Part print with two shaded views. Sizes in mm from the minimum x, y, z corner. A direction names the side the tool comes from. Coordinates: 2 decimals unless noted, no trailing zeros. Order: outer loops, then holes, each group sorted by start corner. A loop starts at its lowest first (then second) coordinate and runs counter-clockwise, first axis right, second up. Notation, with made-up numbers: (8.25, 89.25) - (39.25, 89.25) arc R19 cw to (39.25, 115.25) - close; hole circle Ø9 at (73, 49). An arc over 180 degrees is marked (long way). Return JSON: item names as keys, results as strings.
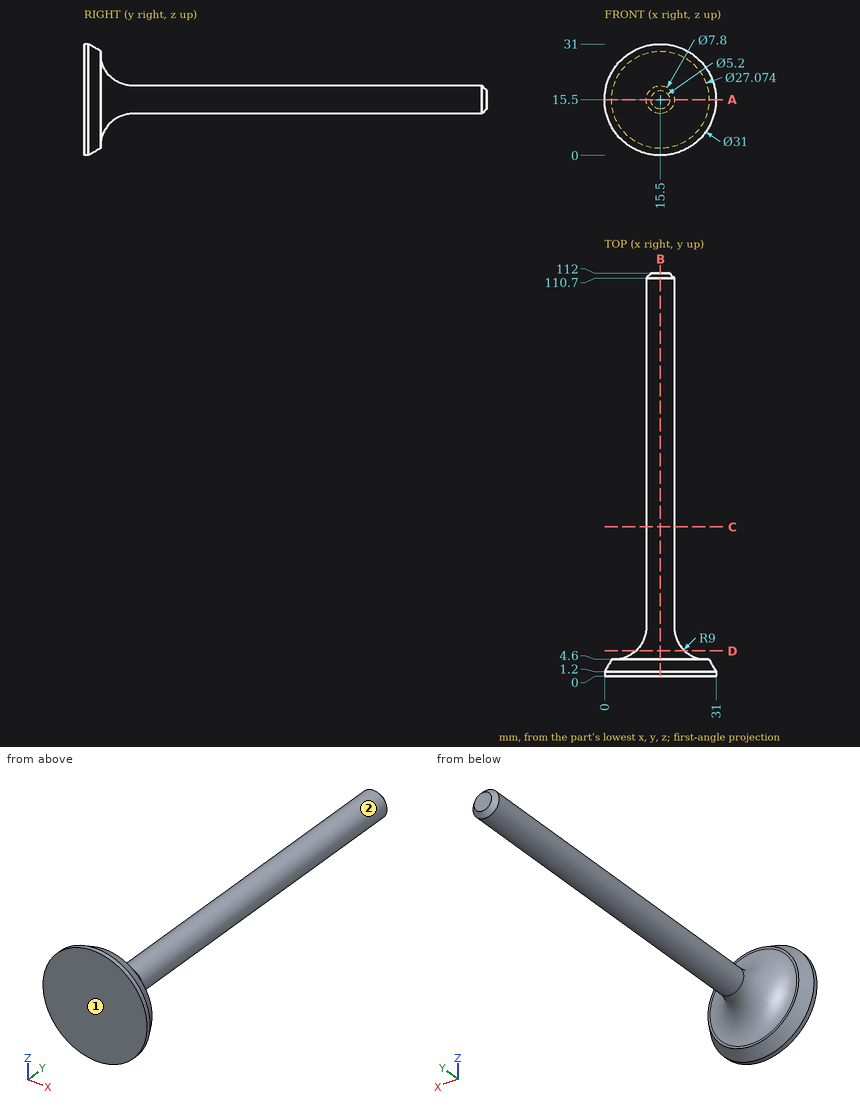
Item 1: Which spindle directions (+Z, -Z, +X, -X, +Y, -Y) get a long thin tool onto all of the face, cutting with end or side? Do the marked faces 1 and 2. Say none if no direction does.
Findings below:
{"face 1": "+Z, -Z, +X, -X, -Y", "face 2": "+Y"}
Item 2: Drop flat-ended pins along their axis: P1, Ø1.5, axis at x = 12, z = 7, coming from the +Y side; P2, Ø12, axis at x = 13, y = 21, coming from the -Z side; P3, Ø3, axis at x = 15.5, z = 10.5, coming from the +Y side; P4, Ø4, axis at y = 94.5, z = 9.5, coming from the +X side. Give the stop position or say it passes through.
Findings below:
{"P1": "stops at y = 5.78", "P2": "stops at z = 11.6", "P3": "stops at y = 111.1", "P4": "passes through"}
Item 3: Band-saw the part on B-B, the plane x = 15.5. List the corners of the cut face in (y, z).
Findings below:
{"outline": "(0, 0) - (1.2, 0) - (4.6, 1.96) - (4.6, 2.6) arc R9 cw to (13.6, 11.6) - (110.7, 11.6) - (112, 12.9) - (112, 18.1) - (110.7, 19.4) - (13.6, 19.4) arc R9 cw to (4.6, 28.4) - (4.6, 29.04) - (1.2, 31) - (0, 31) - close"}
Item 4: Band-saw the part on C-C, the plane y = 41.5. List the corners of the cut face in (x, z), then the cut area to 3 significant figures.
Findings below:
{"outline": "circle Ø7.8 at (15.5, 15.5)", "area": "47.8 mm²"}
Item 5: Wall check: L1, parallel to Y at x = 3, z = 19.5; L2, parallel to Y at x = 14.5, z = 26; L3, parallel to X at y = 61, z = 18. Give the ranges that are in metal, low to high. Write a range as [from, to].
Findings below:
{"L1": "y = [0, 4.6]", "L2": "y = [0, 4.91]", "L3": "x = [12.51, 18.49]"}
Item 6: Band-saw the part on D-D, the plane y = 7. List the corners of the cut face in (x, z).
Findings below:
{"outline": "circle Ø13.56 at (15.5, 15.5)"}
Item 7: Band-saw the part on A-A, the plane z = 15.5. List the corners of the cut face in (x, y).
Findings below:
{"outline": "(0, 0) - (31, 0) - (31, 1.2) - (29.04, 4.6) - (28.4, 4.6) arc R9 cw to (19.4, 13.6) - (19.4, 110.7) - (18.1, 112) - (12.9, 112) - (11.6, 110.7) - (11.6, 13.6) arc R9 cw to (2.6, 4.6) - (1.96, 4.6) - (0, 1.2) - close"}
